Input: dimensioned drawing with shaded views. Units: mm. Origin: part minimum x, y, z. A direction names the side the tool comes from. Give positions to 0.01 mm unless a question says otherwise; leave off trailing zeros. Order: outer loops, then holes, each group sorted by start corner. A loop starts at its lowest first (then second) coordinate and runs counter-clockwise, first axis right, second up. Notation, with made-up numbers: M 51,29.25 L 56,29.25 A35 ccw 56,64.25 Z; hole C 40.5,-37 d11. An arc over 180 degrees is marked long. Answer in a Markdown table with one row per item. Add a question column.
(1) Material intervals for line 1 along X through (y, z) = (250, 14.5); line 2 along Y through (x, z) = (8, 40), sorted ascending.
(2) Set-up query: the marked faces 1, 2, 3, 4 and 5. Return all of +Z, -Z, +X, -X, +Y, -Y with unobstructed straight access to the full face (end or side cutting, diameter ignored); none if empty.
(3) Section query A-A, the plane z = 25. Return loops of the section in (x, y), plus the area to 3 significant figures.
(4) Pin query (flat end, axial travel): P1, Ø8, axis at y = 219.5, z = 19, coming from the -X side; P2, Ø1.5, axis at x = 8, y = 96.5, coming from the +Z side; P3, Ø15, axis at x = 28.5, y = 237, coming from the +Z side; P4, Ø24, axis at x = 22, y = 162, coming from the -Z side. Return the tip coordinate at first contact, or that it passes through.
(5) Section query D-D, the plane y = 41. Return loops of the section in (x, z).
(6) Section query B-B, the plane x = 25. Return loops of the section in (y, z), plus the area to 3 significant figures.
(7) Section query C-C, the plane y = 136.5. Return loops of the section in (x, z).
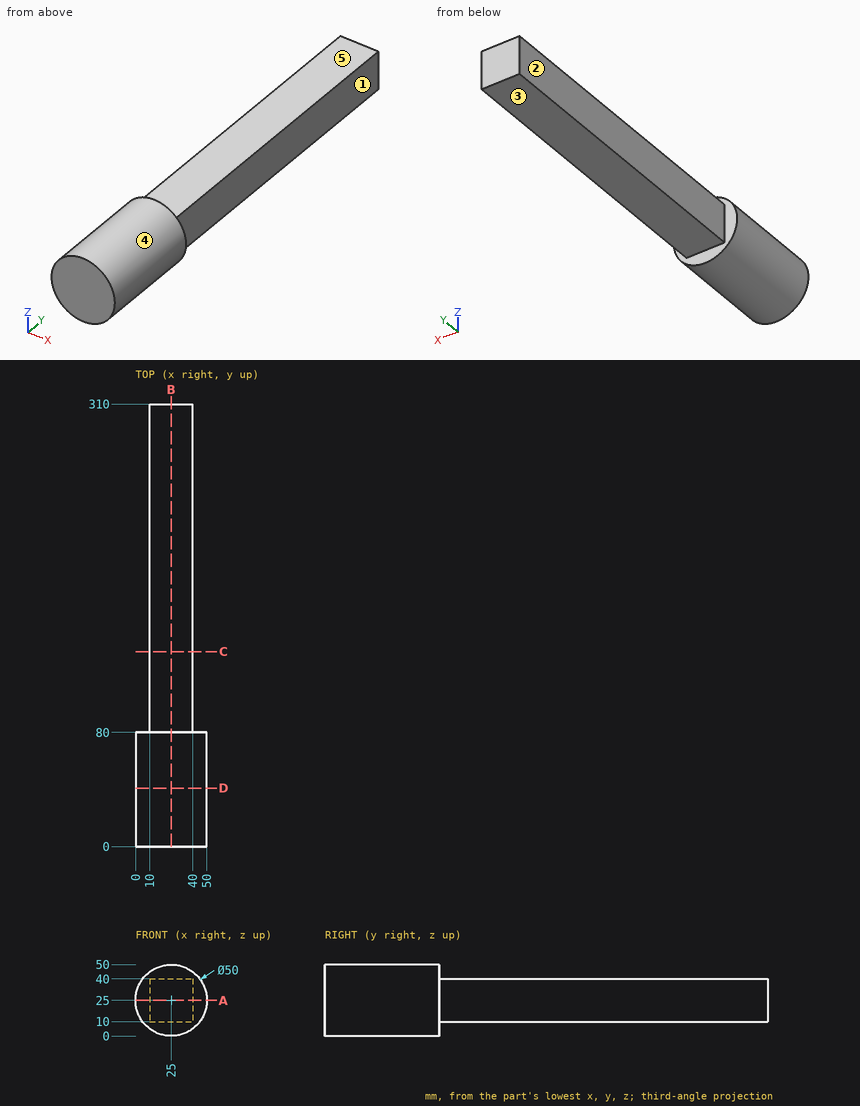
Values follow:
| question | item | result |
|---|---|---|
| 1 | line 1 | x = 10 to 40 |
| 1 | line 2 | y = 0 to 80 |
| 2 | face 1 | +Z, -Z, +X, +Y |
| 2 | face 2 | +Z, -Z, -X, +Y |
| 2 | face 3 | -Z, +X, -X, +Y |
| 2 | face 4 | +Y, -Y |
| 2 | face 5 | +Z, +X, -X, +Y |
| 3 | outline | M 0,0 L 50,0 L 50,80 L 40,80 L 40,310 L 10,310 L 10,80 L 0,80 Z |
| 3 | area | 10,900 mm² |
| 4 | P1 | stops at x = 10 |
| 4 | P2 | passes through |
| 4 | P3 | stops at z = 40 |
| 4 | P4 | stops at z = 10 |
| 5 | outline | C 25,25 d50 |
| 6 | outline | M 0,0 L 80,0 L 80,10 L 310,10 L 310,40 L 80,40 L 80,50 L 0,50 Z |
| 6 | area | 10,900 mm² |
| 7 | outline | M 10,10 L 40,10 L 40,40 L 10,40 Z |
